Part model, mm, in its own coordinate system. Face numbers are marked on the shaded views. A direction names the side the tool comes from. Coordinates: 2 decimals unless noted, no trailing zeros. Write each loop counter-clockwise with the first axis right and the second up, starting at its lowest first coordinate (ties: lowest second). Pieces come first, ordered by that corner, then holes. Notation, with made-up numbers: (64, -17.5) - (71, -17.5) arc R31 ccw to (71, 18.5) - close; hole circle Ø10 at (-33.5, -3.75). An arc over 180 degrees is marked (long way). Use a Markdown table: item, result.
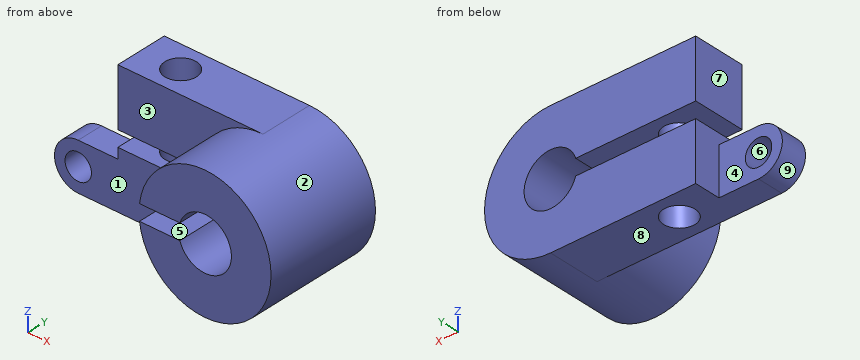
```python
from build123d import *

# Parameters (mm, degrees)
BOSS_EXTRUDE1_DEPTH = 10
BOSS_EXTRUDE2_DEPTH = 45
SKETCH3_R           = 5
BOSS_EXTRUDE3_DEPTH = 10
HOLE1_D             = 12


with BuildPart() as part:
    # Sketch1 → Boss-Extrude1 (new, symmetric)
    with BuildSketch(Plane(origin=(0, 0, 0), x_dir=(1, 0, 0), z_dir=(0, 1, 0))):
        with BuildLine():
            Line((0, 25), (-55, 25))
            Line((-55, 25), (-55, 3))
            Line((-55, 3), (-9.539392014, 3))
            ThreePointArc((-9.539392014, 3), (10, 0), (-9.539392014, -3))
            Line((-9.539392014, -3), (-55, -3))
            Line((-55, -3), (-55, -25))
            Line((-55, -25), (0, -25))
            ThreePointArc((0, -25), (25, 0), (0, 25))
        make_face()
    extrude(amount=BOSS_EXTRUDE1_DEPTH, both=True)

    # Sketch2 → Boss-Extrude2 (add)
    with BuildSketch(Plane(origin=(0, 10, 0), x_dir=(1, 0, 0), z_dir=(0, 1, 0))):
        with BuildLine():
            Line((-9.539392014, -3), (-24.819347292, -3))
            ThreePointArc((-24.819347292, -3), (25, 0), (-24.819347292, 3))
            Line((-24.819347292, 3), (-9.539392014, 3))
            ThreePointArc((-9.539392014, 3), (10, 0), (-9.539392014, -3))
        make_face()
    extrude(amount=-BOSS_EXTRUDE2_DEPTH)

    # Sketch3 → Boss-Extrude3 (add)
    with BuildSketch(Plane.XZ.offset(10)):
        with BuildLine():
            Line((-55, -7), (-70, -7))
            ThreePointArc((-70, -7), (-79, -16), (-70, -25))
            Line((-70, -25), (-55, -25))
            Line((-55, -25), (-55, -7))
        make_face()
        with Locations(Location((-70, -16, 0), (0, 0, 270))):
            Circle(SKETCH3_R, mode=Mode.SUBTRACT)
    extrude(amount=-BOSS_EXTRUDE3_DEPTH)

    # Hole1 (through all)
    with Locations(Plane(origin=(0, 0, -25), x_dir=(-1, 0, 0), z_dir=(0, 0, -1))):
        with Locations((40, 0)):
            Hole(HOLE1_D / 2)


solid = part.part
```
Item 1: Drop flat-ended pins along their axis: P1, Ø3, axis at x = -59, y = -6, coming from the +Z side; P2, Ø16, axis at y = -1, z = 17, coming from the -X side; P3, Ø4, axis at y = 3.5, z = -12, coming from the +X side. Give the stop position or say it passes through.
From the geometry:
| item | result |
|---|---|
| P1 | z = -7 |
| P2 | x = -55 |
| P3 | x = 22.91 |
Item 2: Two-plate mould, pull along Z, no slides. Class the marked faces 6, 7, 8 and 9: pulls with the +Z half, pulls with the -Z half, needs draft (parallel to the pull), parting line crosses it, or undercut.
From the geometry:
| item | result |
|---|---|
| face 6 | undercut |
| face 7 | needs draft |
| face 8 | pulls with the -Z half |
| face 9 | parting line crosses it |
Item 3: Which spindle directions (+Z, -Z, +X, -X, +Y, -Y) get a long thin tool onto all of the face, cutting with end or side? Do the marked faces 1, 2, 3, 4 and 5. Say none if no direction does.
From the geometry:
| item | result |
|---|---|
| face 1 | -Z, -X, -Y |
| face 2 | -Y |
| face 3 | +Z, -X, -Y |
| face 4 | +Z, -Z, -X, +Y |
| face 5 | -X, +Y, -Y |
Item 4: Band-saw the part on D-D, the plane z = 14. Give the cut face in (x, y).
From the geometry:
| item | result |
|---|---|
| outline | (-55, -10) - (-20.71, -10) - (-20.71, -35) - (20.71, -35) - (20.71, 10) - (-55, 10) - close; hole circle Ø12 at (-40, 0) |
Item 5: Band-saw the part on C-C, the plane z = -16. Give the cut face in (x, y), then the cut area to 3 significant figures.
From the geometry:
| item | result |
|---|---|
| outline | (-79, -10) - (-75, -10) - (-75, 0) - (-79, 0) - close; (-65, -10) - (-19.21, -10) - (-19.21, -35) - (19.21, -35) - (19.21, 10) - (-55, 10) - (-55, 0) - (-65, 0) - close; hole circle Ø12 at (-40, 0) |
| area | 2,470 mm^2 |
Item 6: Band-saw the part on B-B, the plane x = -15. Give the cut face in (y, z), then the cut area to 3 significant figures.
From the geometry:
| item | result |
|---|---|
| outline | (-35, -20) - (-10, -20) - (-10, -25) - (10, -25) - (10, -3) - (-35, -3) - close; (-35, 3) - (10, 3) - (10, 25) - (-10, 25) - (-10, 20) - (-35, 20) - close |
| area | 1,730 mm^2 |
Item 7: Band-saw the part on A-A, the plane x = -40. Give the cut face in (y, z).
From the geometry:
| item | result |
|---|---|
| outline | (-10, -25) - (-6, -25) - (-6, -3) - (-10, -3) - close; (-10, 3) - (-6, 3) - (-6, 25) - (-10, 25) - close; (6, -25) - (10, -25) - (10, -3) - (6, -3) - close; (6, 3) - (10, 3) - (10, 25) - (6, 25) - close |
Item 8: Drill centre lines: probe 1 along Z at (x, y) = (-23.5, 6); probe 2 along Z at (x, y) = (0, -18); probe 3 along X at (y, z) = (-5, -16). Where is each one in solid material? Low to high.
From the geometry:
| item | result |
|---|---|
| probe 1 | -25 to -3, 3 to 25 |
| probe 2 | -25 to -10, 10 to 25 |
| probe 3 | -79 to -75, -65 to -43.32, -36.68 to 19.21 |
